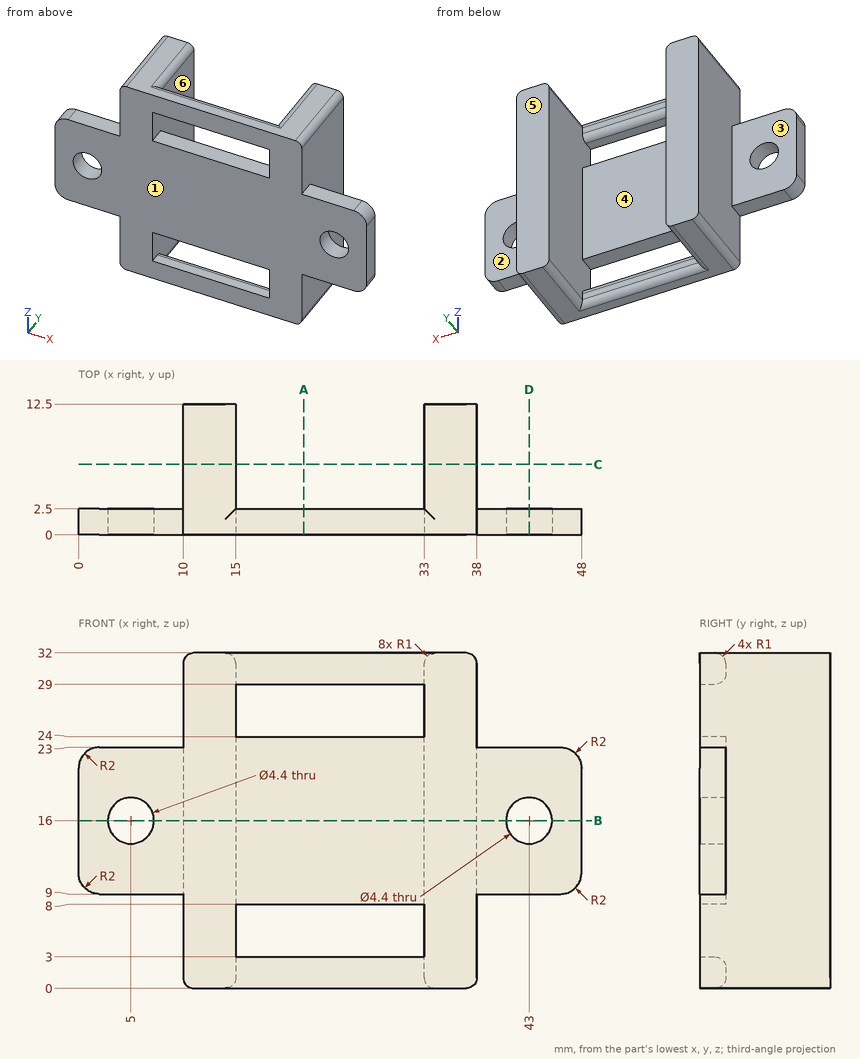
The figure shows three views and two pictorial views of one solid part (mm, origin at its lowest corner). Answer the questions. A direction names the side the tool comes from. Give positions to 0.01 mm unless a question says otherwise; leave off trailing zeros. Write each loop counter-clockwise with the first axis right and the second up, starting at its lowest first coordinate (ties: lowest second). Pieces come first, ordered by that corner, then holes. Notation, with made-up numbers: (32.25, 34) - (50.25, 34) arc R19 cw to (50.25, 51) - close; hole circle Ø4 at (64, 42). An arc over 180 degrees is marked (long way). Use one line per item in the form item = value.
1. A cutting plane is placed at A-A (x = 21.5). Write down the section's boundary in (y, z).
Filled in:
outline = (0, 0) - (1.5, 0) arc R1 ccw to (2.5, 1) - (2.5, 2) arc R1 ccw to (1.5, 3) - (0, 3) - close; (0, 8) - (2.5, 8) - (2.5, 24) - (0, 24) - close; (0, 29) - (1.5, 29) arc R1 ccw to (2.5, 30) - (2.5, 31) arc R1 ccw to (1.5, 32) - (0, 32) - close
2. For the marked faces 1, 2, 3 and 4, determine the directions among +Z, -Z, +X, -X, +Y, -Y from which every point of the face is accessible in a straight line to the end or side of a thin tool.
Filled in:
face_1 = +Z, -Z, +X, -X, -Y
face_2 = +Z, -Z, +X, +Y
face_3 = +Z, -Z, -X, +Y
face_4 = +Z, -Z, +Y
3. Consider L1, parallel to X at y = 1.55, z = 16; L2, parallel to X at y = 5, z = 16.5; L3, parallel to Y at x = 45, z = 19. Determine where each line is inside the solid, lowest interval first.
Filled in:
L1 = 0 to 2.8, 7.2 to 40.8, 45.2 to 48
L2 = 10 to 15, 33 to 38
L3 = 0 to 2.5
4. Determine the mould class of the marked faces 5 and 6 for opening direction X: released by +X, released by -X, zero draft, split by the parting line, or undercut.
Filled in:
face_5 = zero draft
face_6 = undercut
5. A cutting plane is placed at C-C (y = 6.75). Write down the section's boundary in (x, z).
Filled in:
outline = (10, 1) arc R1 ccw to (11, 0) - (14, 0) arc R1 ccw to (15, 1) - (15, 31) arc R1 ccw to (14, 32) - (11, 32) arc R1 ccw to (10, 31) - close; (33, 1) arc R1 ccw to (34, 0) - (37, 0) arc R1 ccw to (38, 1) - (38, 31) arc R1 ccw to (37, 32) - (34, 32) arc R1 ccw to (33, 31) - close
6. Each of these flat-tipped pins is pushed along its axis until it touches: pin 1 Ø0.8 at (x, y) = (6, 1.5) entering from +Z; pin 2 Ø1 at (y, z) = (8, 26) entering from +X; pin 3 Ø0.8 at (x, z) = (26.5, 1.5) entering from +Y. Where does it stop, or does it pass through?
Filled in:
pin_1 = 23
pin_2 = 38
pin_3 = 2.5
7. A cutting plane is placed at D-D (x = 43). Write down the section's boundary in (y, z), and give its area (3 significant figures).
Filled in:
outline = (0, 9) - (2.5, 9) - (2.5, 13.8) - (0, 13.8) - close; (0, 18.2) - (2.5, 18.2) - (2.5, 23) - (0, 23) - close
area = 24.0 mm^2
8. A cutting plane is placed at B-B (z = 16). Write down the section's boundary in (x, y), and give its area (3 significant figures).
Filled in:
outline = (0, 0) - (2.8, 0) - (2.8, 2.5) - (0, 2.5) - close; (7.2, 0) - (40.8, 0) - (40.8, 2.5) - (38, 2.5) - (38, 12.5) - (33, 12.5) - (33, 2.5) - (15, 2.5) - (15, 12.5) - (10, 12.5) - (10, 2.5) - (7.2, 2.5) - close; (45.2, 0) - (48, 0) - (48, 2.5) - (45.2, 2.5) - close
area = 198 mm^2
